Here's how the part is built. I have some questions about the finished solid (model axes, mm). Coordinates: 2 decimals unless noted, no trailing zeros. Write each loop counter-clockwise with the first axis right and the second up, starting at its lowest first coordinate (ties: lowest second). Pieces come first, ordered by that corner, then holes.
Item 1: If we section it at D-D (z = 2): Count the separate pieces of the cut face and the enclosed holes in it, then the cut area to 3 significant figures.
Item 2: If I drill on line 1 (Y direction, x = 30, z = 1.2); line 2 (Y direction, x = 29, z = 1.35); line 3 (Y direction, x = 0, z = 3), over which ranges is the centre line in solid material (lowest first)?
Item 3: If we section it at C-C (x = 30): Please give me the cut outline in (y, z), then the cut area to 3 significant figures.
Item 4: I'm going to push flat-ended pins straight in: pin 1 Ø7 at (x, y) = (-27.5, -23) entering from +Z; pin 2 Ø2 at (y, z) = (-34, 1.5) entering from -X; pin 3 Ø2 at (x, z) = (-21.5, 1) entering from +Y; pin 4 Ø0.6 at (x, z) = (24, 1.5) entering from +Y. Where does each tip first touch, or does it pass through?
Item 5: If we section it at B-B (y = 27.5): Please give me the cut outline in (x, z), then the cut area to 3 significant figures.
Item 6: If we section it at A-A (x = 0): Please give me the cut outline in (y, z).
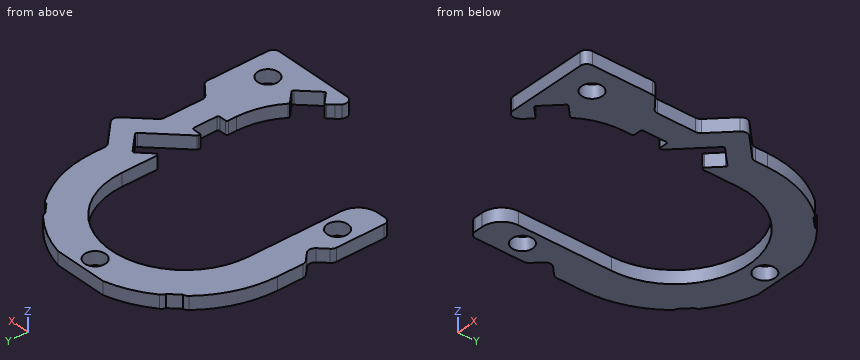
from build123d import *

# Parameters (mm, degrees)
CORPS_DEPTH                     = 4
DIAM_TRE_DU_PER_AGE_6_2_6_3_1_D = 6.3
RENFORT_CAVITE_IR_DEPTH         = 4
CAVITE_IR_DEPTH                 = 73.7636828920554
CAVITE_SWITCH_DEPTH             = 73.7636828920554
CONG_1_R                        = 2
CONG_2_R                        = 0.5


with BuildPart() as part:
    # Esquisse1 → corps (new body)
    with BuildSketch(Plane.XY):
        with BuildLine():
            Line((-21.522272155725624, 24.35069928047194), (-21.522272155725624, 25.01583101267831))
            ThreePointArc((-21.522272155725624, 25.01583101267831), (-15.198873528041206, 29.291538769388826), (-8.062257748298553, 32))
            Line((-8.062257748298553, 32), (8.062257748298553, 32))
            ThreePointArc((8.062257748298553, 32), (15.198873528041206, 29.29153876938882), (21.522272155725624, 25.015831012678305))
            Line((21.522272155725624, 25.015831012678305), (21.522272155725624, 24.350699280471943))
            Line((21.522272155725624, 24.350699280471943), (24.35069928047182, 21.522272155725762))
            Line((24.35069928047182, 21.522272155725762), (25.015831012678188, 21.522272155725762))
            ThreePointArc((25.015831012678188, 21.522272155725762), (30.93963819615851, 11.477751883135042), (33, 0))
            Line((33, 0), (33, -34.48090133377067))
            Line((33, -34.48090133377067), (38, -38.48090133377066))
            Line((38, -38.48090133377066), (38, -59.76396103067893))
            Line((38, -59.76396103067893), (9.515567427896173, -59.76396103067893))
            ThreePointArc((9.515567427896173, -59.76396103067893), (9.973004843675767, -57.46613597206372), (11.275567427896174, -55.51868129902402))
            Line((11.275567427896174, -55.51868129902402), (15.9, -50.9))
            ThreePointArc((15.9, -50.9), (20.78460969082653, -43.597044976101124), (22.500000000000004, -34.98020100629408))
            Line((22.500000000000004, -34.98020100629408), (22.5, 0))
            ThreePointArc((22.5, 0), (1.38e-15, 22.5), (-22.5, 0))
            Line((-22.5, 0), (-22.5, -28.480901333770667))
            ThreePointArc((-22.5, -28.480901333770667), (-24.257359312880713, -32.723542020889944), (-28.499999999999993, -34.48090133377067))
            Line((-28.499999999999993, -34.48090133377067), (-33, -34.48090133377067))
            Line((-33, -34.48090133377067), (-33, 0))
            ThreePointArc((-33, 0), (-30.939638196158512, 11.477751883135037), (-25.015831012678195, 21.522272155725755))
            Line((-25.015831012678195, 21.522272155725755), (-24.35069928047182, 21.52227215572576))
            Line((-24.35069928047182, 21.52227215572576), (-21.522272155725624, 24.35069928047194))
        make_face()
    extrude(amount=CORPS_DEPTH)

    # Diamètre du perçage Ø6.2 (6.3)1 (through all)
    with Locations(Plane.XY.offset(4)):
        with Locations((0, 27.5), (30, -51), (-27.5, -23)):
            Hole(DIAM_TRE_DU_PER_AGE_6_2_6_3_1_D / 2)

    # Esquisse4 → renfort_cavite_IR (add, through all)
    with BuildSketch(Plane.XY):
        Polygon((31.414213562373053, -2.928932188134515), (41.313708498984774, -12.828427124746126), (34.525483399593966, -19.61665222413702), (27.454415587728445, -26.68772003600261), (24.62598846298224, -9.717157287525408), align=None)
    extrude(amount=RENFORT_CAVITE_IR_DEPTH)

    # Esquisse4<4> → cavite_IR (cut, through all)
    with BuildSketch(Plane.XY):
        Polygon((4.3e-16, -34.34314575050794), (24.62598846298224, -9.717157287525408), (27.17157287525379, -7.171572875253825), (32.828427124746206, -12.828427124746176), (30.282842712474658, -15.37401153701776), (1.73e-15, -45.65685424949275), align=None)
        Polygon((-75.93969696196702, -31.797561338236385), (-42.82842712474626, 1.313708498984752), (-28.686291501015212, -12.828427124746126), (-61.79756133823598, -45.93969696196728), align=None)
    extrude(amount=CAVITE_IR_DEPTH, mode=Mode.SUBTRACT)

    # Esquisse5 → cavite_switch (cut, through all)
    with BuildSketch(Plane.XY):
        Polygon((18.90520382004283, -48.24834957055045), (21.910407640085666, -51.25355339059327), (22.263961030678935, -51.607106781186545), (16.607106781186562, -57.26396103067893), (16.253553390593282, -56.910407640085644), (13.24834957055045, -53.905203820042814), (12.894796179957178, -53.551650429449545), (11.671501448504449, -52.32835569799682), (17.32835569799682, -46.671501448504436), (18.55165042944955, -47.89479617995717), align=None)
        Polygon((20.249999999999996, -31.999999999999993), (18.51999999999999, -32), (18.51999999999999, -23.999999999999993), (20.249999999999996, -23.999999999999996), (20.750000000000007, -23.99999999999999), (25.000000000000007, -23.99999999999999), (25.50000000000001, -24), (25.500000000000007, -32), (25.00000000000001, -32), (20.750000000000007, -32), align=None)
    extrude(amount=CAVITE_SWITCH_DEPTH, mode=Mode.SUBTRACT)

    # Congé1
    # the kernel refuses this fillet: 2 mm, written as the material it adds along each edge
    with BuildSketch(Plane(origin=(33, -4.514718625761442, 0), x_dir=(0.7071067811865507, -0.7071067811865442, 0), z_dir=(0, 0, 1))) as cong_1_piece_1:
        with BuildLine():
            CenterArc((CONG_1_R * 0.414213562373, CONG_1_R), CONG_1_R, 224.99999999999966, 45.000000000000455)
            Line((-CONG_1_R * 0.292893218813, CONG_1_R * 0.292893218813), (0, 0))
            Line((0, 0), (CONG_1_R * 0.414213562373, 1e-17))
        make_face()
    extrude(amount=4)
    with BuildSketch(Plane(origin=(33, -21.142135623731004, 4), x_dir=(0, -1, 0), z_dir=(0, 0, -1))) as cong_1_piece_2:
        with BuildLine():
            CenterArc((CONG_1_R * 0.414213562373, -CONG_1_R), CONG_1_R, 90, 44.999999999999574)
            Line((-CONG_1_R * 0.292893218813, -CONG_1_R * 0.292893218813), (0, 0))
            Line((0, 0), (CONG_1_R * 0.414213562373, 0))
        make_face()
    extrude(amount=4)
    with BuildSketch(Plane(origin=(33, -34.48090133377067, 0), x_dir=(0.7808688094430318, -0.6246950475544225, 0), z_dir=(0, 0, 1))) as cong_1_piece_3:
        with BuildLine():
            CenterArc((CONG_1_R * 0.480624847487, CONG_1_R), CONG_1_R, 218.65980825408994, 51.34019174590992)
            Line((-CONG_1_R * 0.300243961956, CONG_1_R * 0.375304952446), (0, 0))
            Line((0, 0), (CONG_1_R * 0.480624847487, 1e-17))
        make_face()
    extrude(amount=4)
    with BuildSketch(Plane(origin=(-28.686291501015212, -12.828427124746126, 0), x_dir=(-0.7071067811865511, 0.707106781186544, 0), z_dir=(0, 0, 1))) as cong_1_piece_4:
        with BuildLine():
            CenterArc((CONG_1_R, CONG_1_R), CONG_1_R, 179.9999999999999, 90.00000000000023)
            Line((-7.52e-15, CONG_1_R), (0, 0))
            Line((0, 0), (CONG_1_R, 2e-17))
        make_face()
    extrude(amount=4)
    # the kernel refuses this fillet: 2 mm, written as the material it takes off along each edge
    with BuildSketch(Plane(origin=(-25.0158310126782, 21.52227215572575, -2.3412126230346395), x_dir=(1, 0, 0), z_dir=(0, 0, 1))) as cong_1_2_piece_1:
        with BuildLine():
            CenterArc((0.9518811347481559, -1.979336954674956), CONG_1_R, 98.24317304928408, 42.67591267968572)
            ThreePointArc((-0.6006317606021696, -0.7185024255749006), (-0.30286474640058003, -0.35712048938501084), (0, 0))
            Line((0, 0), (0.6651317322063797, 0))
        make_face()
    extrude(amount=8.682425246069279, mode=Mode.SUBTRACT)
    with BuildSketch(Plane(origin=(-21.522272155725624, 25.015831012678312, -2.341212623034707), x_dir=(0.7672332048205719, 0.6413682323133525, 0), z_dir=(0, 0, 1))) as cong_1_2_piece_2:
        with BuildLine():
            CenterArc((0.9081067143892164, -1.9997986573934323), CONG_1_R, 89.18699331013795, 42.675912679686405)
            Line((-0.4265943633407193, -0.5103111505285536), (0, 0))
            ThreePointArc((0, 0), (0.46824252460693927, 0.00332215300834937), (0.936485049213883, -9e-17))
        make_face()
    extrude(amount=8.682425246069414, mode=Mode.SUBTRACT)
    with BuildSketch(Plane(origin=(25.015831012678184, 21.522272155725762, -2.341212623034682), x_dir=(0.6413682323133517, -0.7672332048205726, 0), z_dir=(0, 0, 1))) as cong_1_2_piece_3:
        with BuildLine():
            CenterArc((0.9081067143892213, -1.9997986573934339), CONG_1_R, 89.18699331013839, 42.67591267968582)
            Line((-0.42659436334071155, -0.5103111505285509), (0, 0))
            ThreePointArc((0, 0), (0.46824252460693927, 0.00332215300834983), (0.936485049213873, -2e-17))
        make_face()
    extrude(amount=8.682425246069364, mode=Mode.SUBTRACT)
    with BuildSketch(Plane(origin=(21.522272155725624, 25.015831012678305, -2.3412126230346706), x_dir=(5.34e-15, -1, 0), z_dir=(0, 0, 1))) as cong_1_2_piece_4:
        with BuildLine():
            CenterArc((0.9518811347481454, -1.9793369546749575), CONG_1_R, 98.24317304928427, 42.67591267968571)
            ThreePointArc((-0.6006317606021806, -0.7185024255749081), (-0.30286474640058547, -0.3571204893850199), (0, 0))
            Line((0, 0), (0.6651317322063619, 0))
        make_face()
    extrude(amount=8.682425246069341, mode=Mode.SUBTRACT)
    with BuildSketch(Plane(origin=(41.313708498984774, -12.828427124746126, -4.999999999999984), x_dir=(-0.7071067811865427, -0.7071067811865525, 0), z_dir=(0, 0, 1))) as cong_1_2_piece_5:
        with BuildLine():
            CenterArc((CONG_1_R, -CONG_1_R), CONG_1_R, 90.00000000000004, 89.99999999999976)
            Line((-1.126e-14, -CONG_1_R), (0, 0))
            Line((0, 0), (CONG_1_R, -5e-17))
        make_face()
    extrude(amount=13.999999999999968, mode=Mode.SUBTRACT)
    with BuildSketch(Plane(origin=(38, -38.48090133377066, -2.403124237432852), x_dir=(0, -1, 0), z_dir=(0, 0, 1))) as cong_1_2_piece_6:
        with BuildLine():
            CenterArc((CONG_1_R * 0.480624847487, -CONG_1_R), CONG_1_R, 90, 51.340191745909806)
            Line((-CONG_1_R * 0.300243961956, -CONG_1_R * 0.375304952446), (0, 0))
            Line((0, 0), (CONG_1_R * 0.480624847487, 0))
        make_face()
    extrude(amount=8.806248474865704, mode=Mode.SUBTRACT)
    with BuildSketch(Plane(origin=(38, -59.76396103067893, -5), x_dir=(-1, 0, 0), z_dir=(0, 0, 1)), Plane(origin=(-33, -34.48090133377067, -5), x_dir=(0, 1, 0), z_dir=(0, 0, 1))) as cong_1_2_piece_7:
        with BuildLine():
            CenterArc((CONG_1_R, -CONG_1_R), CONG_1_R, 90, 90)
            Line((0, -CONG_1_R), (0, 0))
            Line((0, 0), (CONG_1_R, 0))
        make_face()
    extrude(amount=14, mode=Mode.SUBTRACT)
    with BuildSketch(Plane(origin=(9.515567427896173, -59.76396103067893, -7.764571353075624), x_dir=(1, 0, 0), z_dir=(0, 0, 1))) as cong_1_2_piece_8:
        with BuildLine():
            CenterArc((2.5358983848622465, 2), CONG_1_R, 150, 120)
            ThreePointArc((0.8038475772933698, 3), (0.20444504226559168, 1.5529142706151262), (0, 0))
            Line((0, 0), (2.5358983848622465, 0))
        make_face()
    extrude(amount=19.529142706151248, mode=Mode.SUBTRACT)
    with BuildSketch(Plane(origin=(-33, -17.142135623730965, -2.0710678118654613), x_dir=(0.7071067811865432, 0.7071067811865518, 0), z_dir=(0, 0, 1))) as cong_1_2_piece_9:
        with BuildLine():
            CenterArc((CONG_1_R * 0.414213562373, -CONG_1_R), CONG_1_R, 90.00000000000003, 44.99999999999963)
            Line((-CONG_1_R * 0.292893218813, -CONG_1_R * 0.292893218813), (0, 0))
            Line((0, 0), (CONG_1_R * 0.414213562373, 1e-17))
        make_face()
    extrude(amount=8.142135623730923, mode=Mode.SUBTRACT)
    with BuildSketch(Plane(origin=(-33, -8.51471862576139, 6.071067811865498), x_dir=(0, 1, 0), z_dir=(0, 0, -1))) as cong_1_2_piece_10:
        with BuildLine():
            CenterArc((CONG_1_R * 0.414213562373, CONG_1_R), CONG_1_R, 224.99999999999957, 45.000000000000455)
            Line((-CONG_1_R * 0.292893218813, CONG_1_R * 0.292893218813), (0, 0))
            Line((0, 0), (CONG_1_R * 0.414213562373, 0))
        make_face()
    extrude(amount=8.142135623730995, mode=Mode.SUBTRACT)

    # Congé2
    cong_2_edges = [part.edges().sort_by_distance(p)[0] for p in [
        (22.500000000000007, -11.843145750507656, 2),
        (27.17157287525379, -7.171572875253825, 2),
        (22.500000000000004, -23.15685424949253, 2),
        (32.828427124746206, -12.828427124746176, 2),
        (13.069812964361518, -53.726667213853844, 2),
        (18.47678110683533, -47.81992685734296, 2),
        (22.263961030678935, -51.607106781186545, 2),
        (16.607106781186562, -57.26396103067893, 2),
        (25.50000000000001, -24, 2),
        (22.500000000000004, -31.999999999999986, 2),
        (25.500000000000007, -32, 2),
    ]]
    fillet(cong_2_edges, radius=CONG_2_R)


solid = part.part
Answer list:
1. separate pieces: 1
1. enclosed holes: 3
1. area: 1,930 mm2
2. line 1: y = -59.76 to -54.15, -47.85 to -15.66, -10 to 13.75
2. line 2: y = -59.76 to -53.99, -48.01 to -16.66, -9 to 15.75
2. line 3: y = 22.5 to 24.35, 30.65 to 32
3. outline: (-59.76, 0) - (-54.15, 0) - (-54.15, 4) - (-59.76, 4) - close; (-47.85, 0) - (-15.66, 0) - (-15.66, 4) - (-47.85, 4) - close; (-10, 0) - (13.75, 0) - (13.75, 4) - (-10, 4) - close
3. area: 246 mm2
4. pin 1: stops at z = 4
4. pin 2: stops at x = -32.93
4. pin 3: stops at y = 25.86
4. pin 4: stops at y = 22.17
5. outline: (-18.24, 0) - (-3.15, 0) - (-3.15, 4) - (-18.24, 4) - close; (3.15, 0) - (18.24, 0) - (18.24, 4) - (3.15, 4) - close
5. area: 121 mm2
6. outline: (22.5, 0) - (24.35, 0) - (24.35, 4) - (22.5, 4) - close; (30.65, 0) - (32, 0) - (32, 4) - (30.65, 4) - close
